```python
from build123d import *

# Parameters (mm, degrees)
SKETCH1_R           = 5.5
BOSS_EXTRUDE1_DEPTH = 160.3
SKETCH3_OUTSIDE_W   = 45.21
SKETCH3_OUTSIDE_H   = 45.21
SKETCH3_OUTSIDE_R   = 5
CUT_EXTRUDE2_DEPTH  = 120
SKETCH4_OUTSIDE_W   = 45.21
SKETCH4_OUTSIDE_H   = 45.21
SKETCH4_OUTSIDE_R   = 3.96875
CUT_EXTRUDE3_DEPTH  = 37.57
SKETCH5_OUTSIDE_W   = 45.21
SKETCH5_OUTSIDE_H   = 45.21
SKETCH5_OUTSIDE_R   = 3.97
CUT_EXTRUDE4_DEPTH  = 93.36
SKETCH9_W           = 3
SKETCH9_H           = 27
CUT_EXTRUDE6_DEPTH  = 1
SKETCH11_W          = 3.767354336
SKETCH11_H          = 27
CUT_EXTRUDE7_DEPTH  = 1
SKETCH12_R          = 15.914705016
CUT_EXTRUDE8_DEPTH  = 85.98


with BuildPart() as part:
    # Sketch1 → Boss-Extrude1 (new body)
    with BuildSketch(Plane.XY):
        Circle(SKETCH1_R)
    extrude(amount=BOSS_EXTRUDE1_DEPTH)

    # Sketch3 outside → Cut-Extrude2 (cut)
    with BuildSketch(Plane(origin=(0, 0, 0), x_dir=(-1, 0, 0), z_dir=(0, 0, -1))):
        Rectangle(SKETCH3_OUTSIDE_W, SKETCH3_OUTSIDE_H)
        Circle(SKETCH3_OUTSIDE_R, mode=Mode.SUBTRACT)
    extrude(amount=-CUT_EXTRUDE2_DEPTH, mode=Mode.SUBTRACT)

    # Sketch4 outside → Cut-Extrude3 (cut)
    with BuildSketch(Plane.XY.offset(160.3)):
        Rectangle(SKETCH4_OUTSIDE_W, SKETCH4_OUTSIDE_H)
        Circle(SKETCH4_OUTSIDE_R, mode=Mode.SUBTRACT)
    extrude(amount=-CUT_EXTRUDE3_DEPTH, mode=Mode.SUBTRACT)

    # Sketch5 outside → Cut-Extrude4 (cut)
    with BuildSketch(Plane(origin=(0, 0, 0), x_dir=(-1, 0, 0), z_dir=(0, 0, -1))):
        Rectangle(SKETCH5_OUTSIDE_W, SKETCH5_OUTSIDE_H)
        Circle(SKETCH5_OUTSIDE_R, mode=Mode.SUBTRACT)
    extrude(amount=-CUT_EXTRUDE4_DEPTH, mode=Mode.SUBTRACT)

    # Sketch9 → Cut-Extrude6 (cut)
    with BuildSketch(Plane(origin=(0, 5, 0), x_dir=(1, 0, 0), z_dir=(0, 1, 0))):
        with Locations((0, -106.5)):
            Rectangle(SKETCH9_W, SKETCH9_H)
    extrude(amount=-CUT_EXTRUDE6_DEPTH, mode=Mode.SUBTRACT)

    # Sketch11 → Cut-Extrude7 (cut)
    with BuildSketch(Plane(origin=(0, -5, 0), x_dir=(-1, 0, 0), z_dir=(0, -1, 0))):
        with Locations((0, -106.520343873)):
            Rectangle(SKETCH11_W, SKETCH11_H)
    extrude(amount=-CUT_EXTRUDE7_DEPTH, mode=Mode.SUBTRACT)

    # Sketch12 → Cut-Extrude8 (cut)
    with BuildSketch(Plane(origin=(0, 0, 0), x_dir=(-1, 0, 0), z_dir=(0, 0, -1))):
        Circle(SKETCH12_R)
    extrude(amount=-CUT_EXTRUDE8_DEPTH, mode=Mode.SUBTRACT)


solid = part.part
```
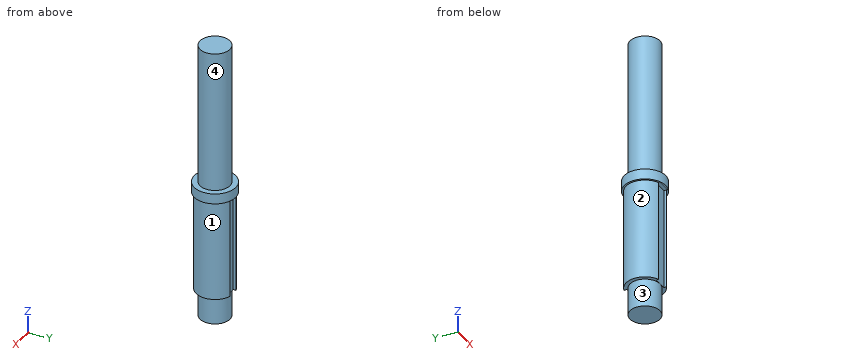
Here's how the part is built. I have some questions about the finished solid (model axes, mm). Face numbers are marked on the shaded views. A direction names the side the tool comes from. Coordinates: 2 decimals unless noted, no trailing zeros. Order: outer loops, then holes, each group sorted by start corner. A loop starts at its lowest first (then second) coordinate and runs counter-clockwise, first axis right, second up.
1) Imagine slicing it at C-C on z = 95.5. List the corners of the cut face in (x, y) for me, and give its area (3 significant figures).
2) Which directions (+Z, -Z, +X, -X, +Y, -Y) give clear straight access to the entire face, cutting with the end or side of a thin tool? Please do the marked faces 1, 2, 3 and 4.
3) Imagine slicing it at B-B on y = 0. List the corners of the cut face in (x, z) for me.
4) Imagine slicing it at D-D on z = 126.5. List the corners of the cut face in (x, y) for me.
5) Will these pins go through, and if not, where does the flat tip stop? pin 1 (1.1 mm diameter, centred on x = 0, z = 110, fed in from -Y); pin 2 (0.6 mm diameter, centred on y = 4.5, z = 107.5, fed in from +X); pin 3 (0.5 mm diameter, centred on y = -4.5, z = 108.5, fed in from -X).
6) I need wall thicknesses on line 1 (X direction, y = -3, z = 103); line 2 (Z direction, x = 2, y = 4.25); line 3 (Z direction, x = 0, y = -5). Which ranges of each line are inside material? Lowest first, please.
Response values:
1. outline: (-1.88, -4.63) - (-1.88, -4) - (1.88, -4) - (1.88, -4.63) arc R5 ccw to (1.5, 4.77) - (1.5, 4) - (-1.5, 4) - (-1.5, 4.77) arc R5 ccw to start
1. area: 72.5 mm2
2. face 1: -Z, +X
2. face 2: -Z, -X
2. face 3: -Z
2. face 4: +Z
3. outline: (-5.5, 120) - (-5, 120) - (-5, 93.36) - (-3.97, 93.36) - (-3.97, 85.98) - (3.97, 85.98) - (3.97, 93.36) - (5, 93.36) - (5, 120) - (5.5, 120) - (5.5, 122.73) - (3.97, 122.73) - (3.97, 160.3) - (-3.97, 160.3) - (-3.97, 122.73) - (-5.5, 122.73) - close
4. outline: circle Ø7.94 at (0, 0)
5. pin 1: stops at y = -4
5. pin 2: stops at x = 2.71
5. pin 3: stops at x = -2.63
6. line 1: x = -4 to 4
6. line 2: z = 93.36 to 122.73
6. line 3: z = 120.02 to 122.73
